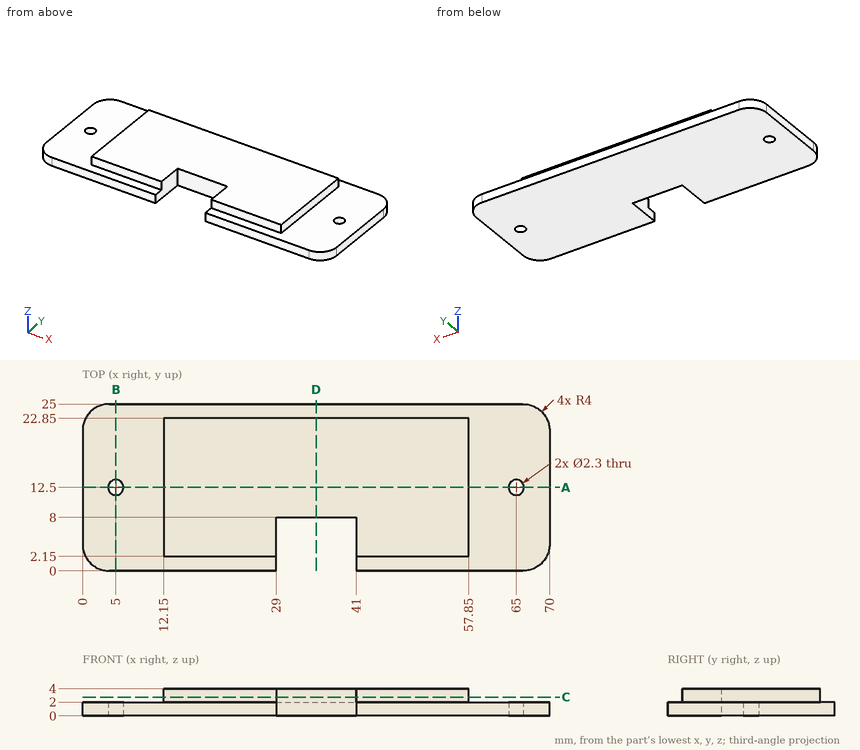
Drawing for the job (mm, zero at the part's lowest x, y, z). Round coordinates to 2 decimals unless told otherwise and drop trailing zeros. Loops run counter-clockwise (first coordinate to the right, second up) from the corner with the lowest first, then second, coordinate; pieces in that order, holes last. Notation, with made-up numbers: (-24, -26) -> (24, -26) arc R20 ccw to (24, -10) -> close; hole circle Ø9 at (-21, 34). An arc over 180 degrees is marked (long way). Use one line per item in the form item = value. Start each with the question number.
Item 1: Band-saw the part on C-C (z = 2.75). List the corners of the cut face in (x, y).
Item 2: Band-saw the part on D-D (x = 35). List the corners of the cut face in (y, z), plus the area to 3 significant figures.
Item 3: Band-saw the part on A-A (y = 12.5). List the corners of the cut face in (x, z), plus the area to 3 significant figures.
Item 4: Drop flat-ended pins along their axis: pin 1 Ø2 at (y, z) = (2.5, 2.5) entering from +X; pin 2 Ø2 at (x, z) = (36.5, 1) entering from -Y; pin 3 Ø1.2 at (y, z) = (4.5, 2.5) entering from -X; pin 4 Ø1 at (x, z) = (49.5, 3) entering from -Y. Give the stop position or say it passes through.
Item 5: Band-saw the part on B-B (x = 5). List the corners of the cut face in (y, z).
Item 6: Drill centre lines: line 1 along Y through (x, z) = (65, 1.5); line 2 along X through (y, z) = (7, 1.7); line 3 along X through (y, z) = (6.25, 3.1). Where is each one in solid material? Low to high.
Data:
q1.outline = (12.15, 2.15) -> (29, 2.15) -> (29, 8) -> (41, 8) -> (41, 2.15) -> (57.85, 2.15) -> (57.85, 22.85) -> (12.15, 22.85) -> close
q2.outline = (8, 0) -> (25, 0) -> (25, 2) -> (22.85, 2) -> (22.85, 4) -> (8, 4) -> close
q2.area = 63.7 mm^2
q3.outline = (0, 0) -> (3.85, 0) -> (3.85, 2) -> (0, 2) -> close; (6.15, 0) -> (63.85, 0) -> (63.85, 2) -> (57.85, 2) -> (57.85, 4) -> (12.15, 4) -> (12.15, 2) -> (6.15, 2) -> close; (66.15, 0) -> (70, 0) -> (70, 2) -> (66.15, 2) -> close
q3.area = 222 mm^2
q4.pin_1 = 69.95
q4.pin_2 = 8
q4.pin_3 = 0
q4.pin_4 = 2.15
q5.outline = (0, 0) -> (11.35, 0) -> (11.35, 2) -> (0, 2) -> close; (13.65, 0) -> (25, 0) -> (25, 2) -> (13.65, 2) -> close
q6.line_1 = 0 to 11.35, 13.65 to 25
q6.line_2 = 0 to 29, 41 to 70
q6.line_3 = 12.15 to 29, 41 to 57.85
